CAD build for the part. Positions are in the model's coordinates, mm. Face numbers are marked on the shaded views. A direction names the side the tool comes from. Coordinates: 2 decimals unless noted, no trailing zeros. Write each loop counter-clockwise with the first axis right and the second up, starting at its lowest first coordinate (ties: lowest second). Pieces come first, ordered by that corner, then holes. Notation, with made-up numbers: (-16.75, 79) - (14.25, 79) arc R14 ccw to (14.25, 103) - close; hole circle Ø8 at (44, 63). An arc over 180 degrees is marked (long way). Answer in a Markdown table with one row per item. Add a question column.
Q1. Drill centre lines: line 1 along X through (y, z) = (76, 10.5); line 2 along Z through (x, y) = (2, 9); line 3 along Y through (x, z) = (52.5, 16). Where is each one in solid material? Low to high. Write a range as from..to.
Q2. Band-saw the part on A-A (x = 81.5). List the corners of the cut face in (y, z), and give its area (3 significant figures).
Q3. Band-saw the part on D-D (y = 9.25). List the corners of the cut face in (x, z).
Q4. Two-plate mould, pull along X, no slides. Class the marked faces 1, 2 and 3: +X half, -X half, draft (parallel to the pull), parting line (faces both ways), or undercut.
Q5. Band-saw the part on C-C (y = 61.5). List the corners of the cut face in (x, z).
Q6. 3-axis set-ups, long thin cutter, end or side, ignore diameter. For the marked faces 4 and 5: which of +Z, -Z, +X, -X, +Y, -Y reach the whole face in a straight line?
Q7. Pin check, flat tips, straight feed: pin 1 (8 mm diameter, centred on x = 146.5, z = 17.5, fed in from -Y); pin 2 (5 mm diameter, centred on x = 28.5, z = 6.5, fed in from +Y); pin 3 (19 mm diameter, centred on x = 64, z = 15.5, fed in from -Y). Stop position of each tip, or through.
Q8. Band-saw the part on B-B (z = 19). List the corners of the cut face in (x, y).
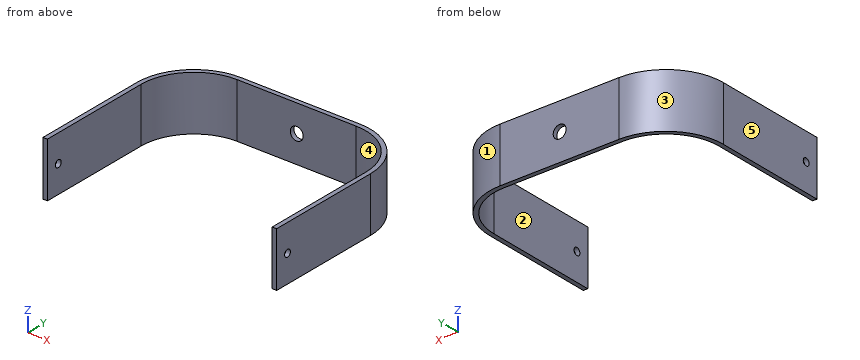
Autodesk Inventor part; units mm, degrees
ref_plane "YZ Plane" through (0, 0, 0) normal (1, 0, 0) x (0, 1, 0)
ref_plane "XZ Plane" through (0, 0, 0) normal (0, 1, 0) x (-1, 0, 0)
ref_plane "XY Plane" through (0, 0, 0) normal (0, 0, 1) x (1, 0, 0)
sketch "Sketch1" plane through (0, 0, 0) normal (0, 0, 1) x (1, 0, 0)
  line L0 (0, 0) -> (0, 80)
  line L1 (163, 0) -> (163, 80)
  line L2 (0, 0) -> (3.1, 0)
  line L3 (3.1, 0) -> (3.1, 80)
  line L4 (163, 0) -> (159.9, 0)
  line L5 (159.9, 0) -> (159.9, 80)
  arc A0 (40, 116.9) -> (3.1, 80) centre (40, 80) ccw
  arc A1 (159.9, 80) -> (123, 116.9) centre (123, 80) ccw
  line L6 (40, 116.9) -> (123, 116.9)
  arc A2 (40, 120) -> (0, 80) centre (40, 80) ccw
  line L7 (40, 120) -> (123, 120)
  arc A3 (163, 80) -> (123, 120) centre (123, 80) ccw
  dimension "d0" = 163
  dimension "d1" = 80
  dimension "d2" = 3.1
  dimension "d3" = 3.1
  dimension "d4" = 3.1
  dimension "d5" = 120
extrude "Extrusion1" add sketch "Sketch1" along normal blind 38
sketch "Sketch2" plane through (163, 0, 0) normal (1, 0, 0) x (0, 0, -1)
  circle A0 centre (-19, 9.25) radius 2.5
  line L0 (-38, 0) -> (-38, 80)
  line L1 (0, 0) -> (-38, 0)
  dimension "d8" = 5
  dimension "d9" = 19
  dimension "d10" = 9.25
extrude "Extrusion2" cut sketch "Sketch2" against normal through all
sketch "Sketch3" plane through (40, 120, 0) normal (0, 1, 0) x (1, 0, 0)
  circle A0 centre (41.5, -19) radius 4.5
  line L0 (-40, 0) -> (-40, -38)
  line L1 (83, 0) -> (0, 0)
  point P0 (-40, -19)
  dimension "d13" = 81.5
  dimension "d14" = 19
  dimension "d15" = 9
extrude "Extrusion3" cut sketch "Sketch3" against normal up to surface (3.1 mm away)
properties part number "pulley_bracket"
Checked values:
| question | item | result |
|---|---|---|
| 1 | line 1 | x = 0..3.1, 159.9..163 |
| 1 | line 2 | z = 0..16.51, 21.49..38 |
| 1 | line 3 | y = 116.9..120 |
| 2 | outline | (116.9, 0) - (120, 0) - (120, 14.5) - (116.9, 14.5) - close; (116.9, 23.5) - (120, 23.5) - (120, 38) - (116.9, 38) - close |
| 2 | area | 89.9 mm² |
| 3 | outline | (0, 0) - (3.1, 0) - (3.1, 16.5) - (0, 16.5) - close; (0, 21.5) - (3.1, 21.5) - (3.1, 38) - (0, 38) - close; (159.9, 0) - (163, 0) - (163, 16.5) - (159.9, 16.5) - close; (159.9, 21.5) - (163, 21.5) - (163, 38) - (159.9, 38) - close |
| 4 | face 1 | +X half |
| 4 | face 2 | undercut |
| 4 | face 3 | -X half |
| 5 | outline | (0, 0) - (3.1, 0) - (3.1, 38) - (0, 38) - close; (159.9, 0) - (163, 0) - (163, 38) - (159.9, 38) - close |
| 6 | face 4 | +Z, -Z, -Y |
| 6 | face 5 | +Z, -Z, -X, +Y, -Y |
| 7 | pin 1 | stops at y = 104.6 |
| 7 | pin 2 | stops at y = 118.97 |
| 7 | pin 3 | stops at y = 116.9 |
| 8 | outline | (0, 0) - (3.1, 0) - (3.1, 6.75) - (0, 6.75) - close; (0, 11.75) - (3.1, 11.75) - (3.1, 80) arc R36.9 cw to (40, 116.9) - (77, 116.9) - (77, 120) - (40, 120) arc R40 ccw to (0, 80) - close; (86, 116.9) - (123, 116.9) arc R36.9 cw to (159.9, 80) - (159.9, 11.75) - (163, 11.75) - (163, 80) arc R40 ccw to (123, 120) - (86, 120) - close; (159.9, 0) - (163, 0) - (163, 6.75) - (159.9, 6.75) - close |
